Source: CAD feature listing. Evaluate the final solid. Frame: model axes, mm. A direction names the side the tool comes from. Give positions to 0.01 mm unless a question says otherwise; leave off trailing zeros. Order: outer loops, then holes, each group sorted by start corner. A loop starts at its lowest first (then second) coordinate and runs counter-clockwise, first axis right, second up.
from build123d import *

# Parameters (mm, degrees)
SKETCH1_W           = 206.5
SKETCH1_H           = 304
SKETCH1_W_2         = 182.5
SKETCH1_H_2         = 280
BOSS_EXTRUDE1_DEPTH = 2
SKETCH2_W           = 206.5
SKETCH2_H           = 304
SKETCH2_W_2         = 196.5
SKETCH2_H_2         = 294
BOSS_EXTRUDE2_DEPTH = 6


with BuildPart() as part:
    # Sketch1 → Boss-Extrude1 (new body)
    with BuildSketch(Plane(origin=(0, 0, 0), x_dir=(1, 0, 0), z_dir=(0, 1, 0))):
        Rectangle(SKETCH1_W, SKETCH1_H)
        Rectangle(SKETCH1_W_2, SKETCH1_H_2, mode=Mode.SUBTRACT)
    extrude(amount=BOSS_EXTRUDE1_DEPTH)

    # Sketch2 → Boss-Extrude2 (add)
    with BuildSketch(Plane(origin=(0, 2, 0), x_dir=(1, 0, 0), z_dir=(0, 1, 0))):
        Rectangle(SKETCH2_W, SKETCH2_H)
        Rectangle(SKETCH2_W_2, SKETCH2_H_2, mode=Mode.SUBTRACT)
    extrude(amount=BOSS_EXTRUDE2_DEPTH)


solid = part.part
(1) Line query: line 1 along Z through (x, y) = (5, 3.75); line 2 along X through (y, z) = (6, -106); line 3 along X through (y, z) = (0.75, 137). Output: solid intervals per line, ascending.
(2) Section B-B, the plane x = 51. Return loops of the section in (y, z), plus the area to 3 significant figures.
(3) Section C-C, the plane y = 6. Return loops of the section in (x, z), plus the area to 4 significant figures.
(4) Section A-A, the plane z = 73.5. Return loops of the section in (x, y), plus the area to 3 significant figures.
(5) Draft query along Z for faces 1 (the flat face through (-103.25, 4, 2)), 2 (the flat face through (98.25, 5, 2)), 3 (the flat face through (-1, 4, -152)). Return one class per face: +Z half, -Z half, draft (parallel to the pull), parting line (faces both ways), or undercut.
(6) Access query for faces 4 (the flat face through (-92, 0, -12)), 5 (the flat face through (-1, 5, 147)). Directions: +Z, -Z, +X, -X, +Y, -Y. A direction counts if a zero-diameter tool reaches every point of the face in a straight line with its end or side. Return the directions, or none.
Checks:
1. line 1: z = -152 to -147, 147 to 152
1. line 2: x = -103.25 to -98.25, 98.25 to 103.25
1. line 3: x = -103.25 to -91.25, 91.25 to 103.25
2. outline: (0, -152) - (8, -152) - (8, -147) - (2, -147) - (2, -140) - (0, -140) - close; (0, 140) - (2, 140) - (2, 147) - (8, 147) - (8, 152) - (0, 152) - close
2. area: 108 mm2
3. outline: (-103.25, -152) - (103.25, -152) - (103.25, 152) - (-103.25, 152) - close; hole (-98.25, -147) - (98.25, -147) - (98.25, 147) - (-98.25, 147) - close
3. area: 5,005 mm2
4. outline: (-103.25, 0) - (-91.25, 0) - (-91.25, 2) - (-98.25, 2) - (-98.25, 8) - (-103.25, 8) - close; (91.25, 0) - (103.25, 0) - (103.25, 8) - (98.25, 8) - (98.25, 2) - (91.25, 2) - close
4. area: 108 mm2
5. face 1: draft
5. face 2: undercut
5. face 3: -Z half
6. face 4: +Z, -Z, +X, -X, -Y
6. face 5: +Y
